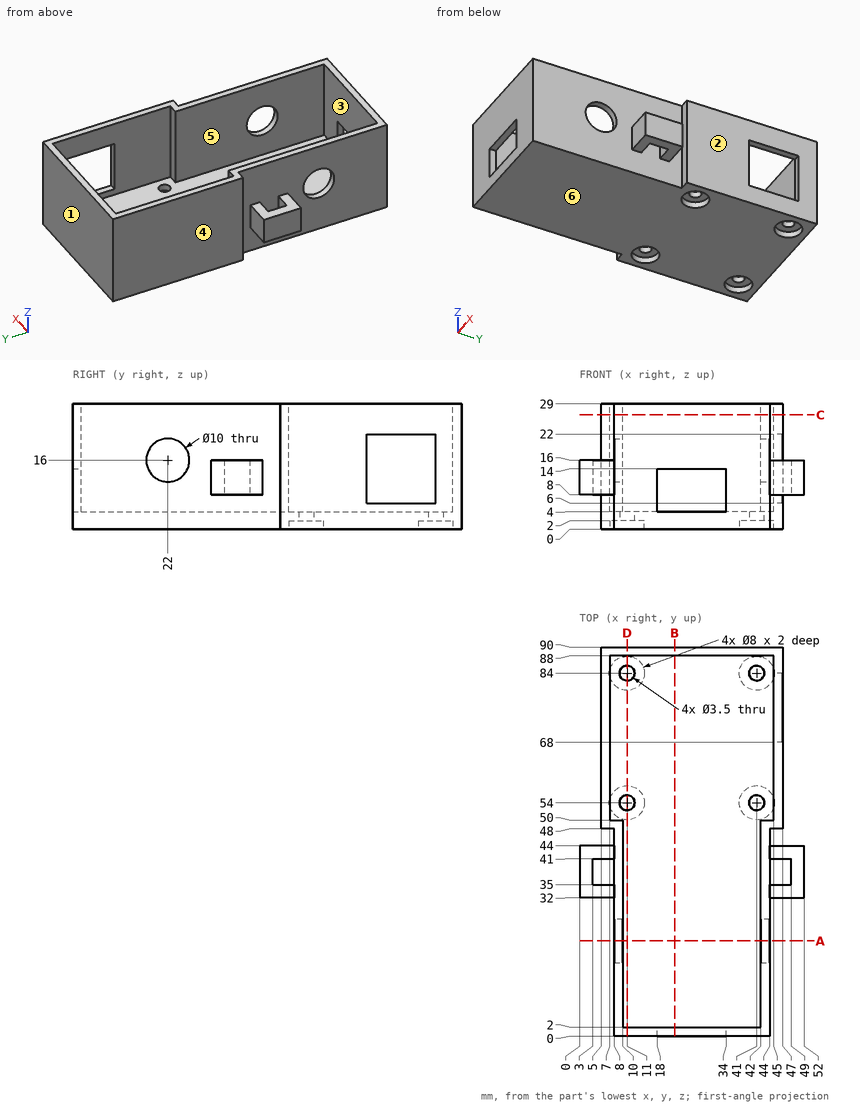
Input: dimensioned drawing with shaded views. Units: mm. Origin: part minimum x, y, z. A direction names the side the tool comes from. Give positions to 0.01 mm unless a question says otherwise; leave off trailing zeros. Order: outer loops, then holes, each group sorted by start corner. A loop starts at its lowest first (then second) coordinate and runs counter-clockwise, first axis right, second up. Notation, with made-up numbers: (-31.5, 46) -> (-5.5, 46) arc R15 cw to (-5.5, 53) -> close; hole circle Ø8 at (-5, 77.5). An arc over 180 degrees is marked (long way). Use a Markdown table: item, result.
1) Section query D-D, the plane x = 11. Return the cut outline in (y, z).
Answer list:
| item | result |
|---|---|
| outline | (0, 0) -> (50, 0) -> (50, 2) -> (52.25, 2) -> (52.25, 4) -> (2, 4) -> (2, 29) -> (0, 29) -> close; (55.75, 2) -> (58, 2) -> (58, 0) -> (80, 0) -> (80, 2) -> (82.25, 2) -> (82.25, 4) -> (55.75, 4) -> close; (85.75, 2) -> (88, 2) -> (88, 0) -> (90, 0) -> (90, 29) -> (88, 29) -> (88, 4) -> (85.75, 4) -> close |
2) Contact query for flat-ended pins moving along their axis: P1, Ø5, axis at x = 32.5, y = 33, coming from the +Z side; P2, Ø3.5, axis at x = 6, z = 7.5, coming from the -Y side; P3, Ø2, axis at x = 25.5, z = 11.5, coming from the -Y side; P4, Ø5, axis at x = 15.5, y = 16, coming from the -Z side. Output: stop coordinate, or through.
Answer list:
| item | result |
|---|---|
| P1 | z = 4 |
| P2 | y = 32 |
| P3 | y = 88 |
| P4 | z = 0 |
3) Reachability of the marked faces 1, 2 and 3 from +Z, -Z, +X, -X, +Y, -Y: full face, straight path, thin tool, end or side. Return the list, or none.
Answer list:
| item | result |
|---|---|
| face 1 | +Z, -Z, +X, -X, +Y |
| face 2 | +Z, -Z, +X, +Y |
| face 3 | +Z |
4) Section query C-C, the plane z = 26.5. Return the cut outline in (x, y).
Answer list:
| item | result |
|---|---|
| outline | (5, 48) -> (8, 48) -> (8, 0) -> (44, 0) -> (44, 48) -> (47, 48) -> (47, 90) -> (5, 90) -> close; hole (7, 50) -> (10, 50) -> (10, 2) -> (42, 2) -> (42, 50) -> (45, 50) -> (45, 88) -> (7, 88) -> close |
5) Ray query, line 1 along X through (y, z) = (84, 1.2); line 2 along Y through (x, z) = (11, 2.55); line 3 along Y through (x, z) = (11, 0.55). Return the intervals inside material, ascending. Write a range as [from, to].
Answer list:
| item | result |
|---|---|
| line 1 | [5, 7], [15, 37], [45, 47] |
| line 2 | [0, 52.25], [55.75, 82.25], [85.75, 90] |
| line 3 | [0, 50], [58, 80], [88, 90] |
6) Section query A-A, the plane y = 22. Return the cut outline in (x, z), then the cut area to 3 significant figures.
Answer list:
| item | result |
|---|---|
| outline | (8, 0) -> (44, 0) -> (44, 11) -> (42, 11) -> (42, 4) -> (10, 4) -> (10, 11) -> (8, 11) -> close; (8, 21) -> (10, 21) -> (10, 29) -> (8, 29) -> close; (42, 21) -> (44, 21) -> (44, 29) -> (42, 29) -> close |
| area | 204 mm² |
7) Mould query, pull axis X, two halves, no side actions, for the marked faces 4, 5 and 6. Classes: +X half, -X half, draft (parallel to the pull), parting line (faces both ways), or undercut.
Answer list:
| item | result |
|---|---|
| face 4 | -X half |
| face 5 | undercut |
| face 6 | draft |
8) Section query B-B, the plane x = 22. Return the cut outline in (y, z).
Answer list:
| item | result |
|---|---|
| outline | (0, 0) -> (90, 0) -> (90, 29) -> (88, 29) -> (88, 4) -> (0, 4) -> close; (0, 14) -> (2, 14) -> (2, 29) -> (0, 29) -> close |
